CAD build for the part. Positions are in the model's coordinates, mm. Face numbers are marked on the shaded views. A direction names the side the tool comes from. Coordinates: 2 decimals unless noted, no trailing zeros. Loops run counter-clockwise (first coordinate to the right, second up) from the corner with the lowest first, then second, coordinate; pieces in that order, holes last. Notation, with made-up numbers: (54.25, 83.25) -> (92.25, 83.25) arc R31 ccw to (92.25, 109.25) -> close; hole circle Ø4 at (55.5, -14.5). An arc over 180 degrees is marked (long way). Write each question's results on one line, items separated by ' | '.
from build123d import *

# Parameters (mm, degrees)
SKETCH2_R           = 2.5
BOSS_EXTRUDE1_DEPTH = 10
CUT_EXTRUDE1_DEPTH  = 6.2
SKETCH4_W           = 11
SKETCH4_H           = 2
BOSS_EXTRUDE2_DEPTH = 7
FILLET1_R           = 0.762


with BuildPart() as part:
    # Sketch2 → Boss-Extrude1 (new body)
    with BuildSketch(Plane.XY.offset(-3838.451709017)):
        with BuildLine():
            Line((13.5, -20), (12.95, -20))
            ThreePointArc((12.95, -20), (9.15, -16.2), (5.35, -20))
            Line((5.35, -20), (4.15, -20))
            ThreePointArc((4.15, -20), (5.457255271, -16.629000688), (8.695454545, -15.020704023))
            ThreePointArc((8.695454545, -15.020704023), (9.019274473, -14.859874356), (9.15, -14.522774425))
            Line((9.15, -14.522774425), (9.15, 1.95))
            Line((9.15, 1.95), (30.85, 1.95))
            Line((30.85, 1.95), (30.85, -14.522774425))
            ThreePointArc((30.85, -14.522774425), (30.980725527, -14.859874356), (31.304545455, -15.020704023))
            ThreePointArc((31.304545455, -15.020704023), (34.542744729, -16.629000688), (35.85, -20))
            Line((35.85, -20), (34.65, -20))
            ThreePointArc((34.65, -20), (30.85, -16.2), (27.05, -20))
            Line((27.05, -20), (26.5, -20))
            ThreePointArc((26.5, -20), (26.146446609, -20.146446609), (26, -20.5))
            Line((26, -20.5), (26, -26.452543058))
            Line((26, -26.452543058), (20, -26.452543058))
            Line((20, -26.452543058), (14, -26.452543058))
            Line((14, -26.452543058), (14, -20.5))
            ThreePointArc((14, -20.5), (13.853553391, -20.146446609), (13.5, -20))
        make_face()
        with Locations((20, -20)):
            Circle(SKETCH2_R, mode=Mode.SUBTRACT)
    extrude(amount=BOSS_EXTRUDE1_DEPTH)

    # Sketch3 → Cut-Extrude1 (cut)
    with BuildSketch(Plane.XY.offset(-3828.451709017)):
        Polygon((20, -25.484827557), (24.75, -22.742413779), (24.75, -17.257586221), (20, -14.515172443), (15.25, -17.257586221), (15.25, -22.742413779), align=None)
    extrude(amount=-CUT_EXTRUDE1_DEPTH, mode=Mode.SUBTRACT)

    # Sketch4 → Boss-Extrude2 (add)
    with BuildSketch(Plane(origin=(0, 1.95, 0), x_dir=(1, 0, 0), z_dir=(0, 1, 0))):
        with Locations((20, 3833.451709017)):
            Rectangle(SKETCH4_W, SKETCH4_H)
    extrude(amount=BOSS_EXTRUDE2_DEPTH)

    # Fillet1
    fillet1_edges = [part.edges().sort_by_distance(p)[0] for p in [
        (25.5, 8.95, -3833.451709017),
        (14.5, 8.95, -3833.451709017),
    ]]
    fillet(fillet1_edges, radius=FILLET1_R)


solid = part.part
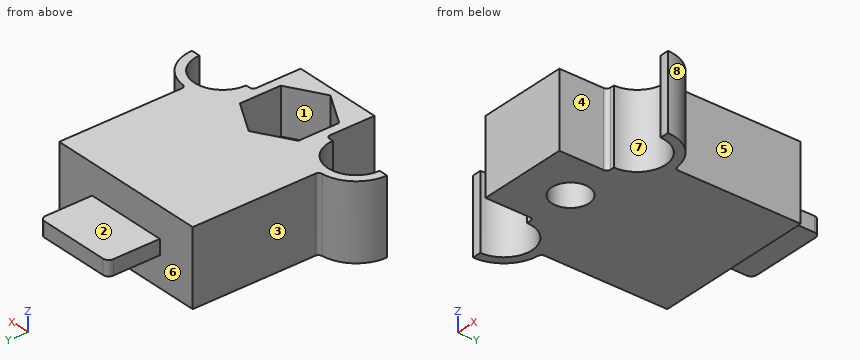
1) Drill centre lines: L1, parallel to Y at x = 20, z = -3836.85; L2, parallel to X at y = -17, z = -3829; L3, parallel to Z at x = 20, y = 4.5. Where is each one in solid material? Low to high. Write a range as from..to.
Outcome:
L1: y = -26.45..-22.5, -17.5..1.95 | L2: x = 5.15..6.82, 11.48..15.7, 24.3..28.52, 33.18..34.85 | L3: z = -3834.45..-3832.45
2) Pin check, flat tips, straight feed: pin 1 (2 mm diameter, centred on x = 21, y = -20, fed in from -Z); pin 2 (3 mm diameter, centred on y = -7, z = -3835.5, fed in from -X); pin 3 (0.6 mm diameter, centred on y = 4, z = -3833, fed in from +X); pin 4 (3 mm diameter, centred on x = 12.5, z = -3831.5, fed in from +Y). Stop position of each tip, or through.
Outcome:
pin 1: passes through | pin 2: stops at x = 9.15 | pin 3: stops at x = 25.5 | pin 4: stops at y = 1.95
3) Slice it at A-A (y = -21.5). Write the cut outline in (x, z), then the cut area to 3 significant figures.
Outcome:
outline: (14, -3838.45) -> (18, -3838.45) -> (18, -3834.65) -> (15.25, -3834.65) -> (15.25, -3828.45) -> (14, -3828.45) -> close; (22, -3838.45) -> (26, -3838.45) -> (26, -3828.45) -> (24.75, -3828.45) -> (24.75, -3834.65) -> (22, -3834.65) -> close | area: 45.9 mm^2
4) Which spindle directions (+Z, -Z, +X, -X, +Y, -Y) get a long thin tool onto all of the face, cutting with end or side? Do the marked faces 1, 2, 3, 4 and 5. Say none if no direction does.
Outcome:
face 1: +Z | face 2: +Z, +X, -X, +Y | face 3: +Z, -Z, -X, +Y | face 4: +Z, -Z, +X, -Y | face 5: +Z, -Z, +X, +Y
5) Slice it at C-C (y = -11). Write the cut outline in (x, z).
Outcome:
outline: (9.15, -3838.45) -> (30.85, -3838.45) -> (30.85, -3828.45) -> (9.15, -3828.45) -> close
6) Two-plate mould, pull along X, no slides. Class the marked faces 6, 7 and 8: pulls with the +X half, pulls with the -X half, needs draft (parallel to the pull), parting line crosses it, or undercut.
Outcome:
face 6: needs draft | face 7: undercut | face 8: pulls with the +X half
7) Slice it at D-D (x = 23). Write the cut outline in (y, z).
Outcome:
outline: (-26.45, -3838.45) -> (1.95, -3838.45) -> (1.95, -3834.45) -> (8.95, -3834.45) -> (8.95, -3832.45) -> (1.95, -3832.45) -> (1.95, -3828.45) -> (-16.25, -3828.45) -> (-16.25, -3834.65) -> (-23.75, -3834.65) -> (-23.75, -3828.45) -> (-26.45, -3828.45) -> close
8) Slice it at B-B (z = -3831.75). Write the cut outline in (x, y).
Outcome:
outline: (4.15, -20) -> (5.35, -20) arc R3.8 cw to (12.95, -20) -> (13.5, -20) arc R0.5 cw to (14, -20.5) -> (14, -26.45) -> (26, -26.45) -> (26, -20.5) arc R0.5 cw to (26.5, -20) -> (27.05, -20) arc R3.8 cw to (34.65, -20) -> (35.85, -20) arc R5 ccw to (31.3, -15.02) arc R0.5 cw to (30.85, -14.52) -> (30.85, 1.95) -> (9.15, 1.95) -> (9.15, -14.52) arc R0.5 cw to (8.7, -15.02) arc R5 ccw to start; hole (15.25, -22.74) -> (20, -25.48) -> (24.75, -22.74) -> (24.75, -17.26) -> (20, -14.52) -> (15.25, -17.26) -> close
